Build history of the part. All positions in model axes, mm. Face numbers are marked on the shaded views. A direction names the side the tool comes from. Give positions to 0.01 mm unless a question says otherwise; leave off trailing zeros. Loops run counter-clockwise (first coordinate to the right, second up) from the corner with the lowest first, then second, coordinate; pieces in that order, holes last. Notation, with made-up numbers: (57, 10.5) -> (111, 10.5) arc R24 cw to (111, 28.5) -> close; hole circle Ø10 at (-26.5, 49.5). An arc over 180 degrees is marked (long way). Answer as a JSON object with one key per item and string values. Group by question number.
Q1. Two-plate mould, pull along Z, no slides. Class the marked faces 5, 6 and 7: pulls with the +Z half, pulls with the -Z half, needs draft (parallel to the pull), parting line crosses it, or undercut.
Q2. Band-saw the part on D-D, the plane y = 7.5. Write the cut outline in (x, z), plus the area to 3 significant figures.
Q3. Band-saw the part on A-A, the plane y = 23. Write the cut outline in (x, z).
Q4. Band-saw the part on C-C, the plane z = -8. Write the cut outline in (x, y).
Q5. Drop flat-ended pins along their axis: pin 1 (3 mm diameter, centred on y = 15.5, z = 6.5, fed in from -X); pin 2 (9 mm diameter, centred on x = 4, y = 13.5, fed in from -Z); pin 3 (3 mm diameter, centred on y = 9, z = -2, fed in from +X). Give the stop position or say it passes through.
Q6. Tool access for the marked faces 1, 2, 3 and 4: list every direction of +Z, -Z, +X, -X, +Y, -Y with a clear straight run to the whole face (end or side of a thin tool).
Q7. Band-saw the part on B-B, the plane x = 0. Write the cut outline in (y, z).
Q8. Wall check: probe 1 along Z at (x, y) = (-7.25, 7.5); probe 2 along Z at (x, y) = (0, 8.5); probe 3 along Z at (x, y) = (-8.5, 5). Give the ranges that are in metal, low to high. Write a range as from..to.
Autodesk Inventor part; units mm, degrees
ref_plane "РабПлоскость1" through (0, 0, 11.75) normal (0, 0, 1) x (1, 0, 0)
ref_plane "YZ Plane" through (0, 0, 0) normal (1, 0, 0) x (0, 1, 0)
ref_plane "XZ Plane" through (0, 0, 0) normal (0, 1, 0) x (-1, 0, 0)
sketch "Эскиз1" plane through (0, 0, 0) normal (0, 1, 0) x (-1, 0, 0)
  circle A0 centre (0, 0) radius 11.75
  dimension "d0" = 23.5
extrude "Выдавливание1" add sketch "Эскиз1" along normal blind 18
sketch "Эскиз2" plane through (0, 0, 0) normal (0, -1, 0) x (1, 0, 0)
  circle A0 centre (0, 0) radius 14
  dimension "d3" = 28
extrude "Выдавливание2" add sketch "Эскиз2" along normal blind 2
sketch "Эскиз3" plane through (0, 18, 0) normal (0, 1, 0) x (1, 0, 0)
  line L0 (0, 11.75) -> (0, -11.75) construction
  line L1 (-0.6, 11.7347) -> (-0.6, 2.4269)
  line L2 (0.6, 11.7347) -> (0.6, 2.4269)
  line L3 (-11.75, 0) -> (11.75, 0) construction
  line L4 (-0.6, -11.7347) -> (-0.6, -2.4269)
  line L5 (0.6, -11.7347) -> (0.6, -2.4269)
  arc A0 (-0.6, 2.4269) -> (-0.6, -2.4269) centre (0, 0) ccw
  arc A1 (0.6, -2.4269) -> (0.6, 2.4269) centre (0, 0) ccw
  circle A2 centre (0, 0) radius 11.75
  line L6 (-11.3865, 2.9) -> (-4.75, 2.9)
  line L7 (-4.75, 2.9) -> (-4.75, -2.9)
  line L8 (-4.75, -2.9) -> (-11.3865, -2.9)
  line L9 (-7.75, 1.9) -> (-5.75, 1.9)
  line L10 (-5.75, 1.9) -> (-5.75, -1.9)
  line L11 (-5.75, -1.9) -> (-7.75, -1.9)
  line L12 (-7.75, -1.9) -> (-7.75, 1.9)
  dimension "d7" = 1.2
  dimension "d8" = 2.5
  dimension "d12" = 5.8
  dimension "d13" = 7
  dimension "d14" = 1
  dimension "d15" = 1
  dimension "d16" = 1
  dimension "d17" = 2
extrude "Выдавливание3" add sketch "Эскиз3" along normal blind 7 contours A2 L2 A1 L5 L4 A0 L1 | L6 L7 L8 A2
sketch "Эскиз4" plane through (0, -2, 0) normal (0, -1, 0) x (1, 0, 0)
  circle A0 centre (0, 0) radius 10.5
  dimension "d18" = 21
extrude "Выдавливание4" cut sketch "Эскиз4" against normal blind 18
sketch "Эскиз5" plane through (0, 0, 0) normal (0, 1, 0) x (1, 0, 0)
  arc A0 (0.6, -11.7347) -> (0.6, 11.7347) centre (0, 0) ccw
  line L0 (11.7155, 0.9) -> (12.95, 0.9)
  line L1 (12.95, 0.9) -> (12.95, -0.9)
  line L2 (12.95, -0.9) -> (11.7155, -0.9)
  line L3 (0, 0) -> (19.973, 0) construction
  point P0 (11.75, 0)
  point P1 (11.75, 0)
  dimension "d21" = 1.8
  dimension "d22" = 1.2
extrude "Выдавливание5" add sketch "Эскиз5" along normal blind 8
chamfer "Фаска1" distance 1.7 angle 35 1 edges at (12.95, 8, 0) measured on face at (12.95, 2.6667, -0.3)
ref_plane "РабПлоскость1" through (0, 0, 11.75) normal (0, 0, 1) x (1, 0, 0)
sketch "Эскиз7" plane through (0, 0, 11.75) normal (0, 0, 1) x (1, 0, 0)
  line L0 (11.75, 18) -> (0.6, 18)
  line L1 (-0.6, 18) -> (-11.3865, 18)
  line L2 (0, 18) -> (4.5, 18)
  line L3 (4.5, 18) -> (4.5, 16)
  line L4 (4.5, 0) -> (0, 0)
  line L5 (14, 0) -> (-14, 0)
  line L6 (0.6, 18) -> (-0.6, 18) construction
  line L7 (0, 18) -> (0, 0) construction
  line L8 (4.5, 0) -> (9.9502, 2.6511)
  line L9 (10.613, 4.7144) -> (4.5, 16)
  arc A0 (9.9502, 2.6511) -> (10.613, 4.7144) centre (9.2941, 4) ccw
  line L10 (0, 18) -> (-4.5, 18)
  line L11 (-4.5, 18) -> (-4.5, 16)
  line L12 (-4.5, 0) -> (0, 0)
  line L13 (-4.5, 0) -> (-9.9502, 2.6511)
  line L14 (-10.613, 4.7144) -> (-4.5, 16)
  arc A1 (-10.613, 4.7144) -> (-9.9502, 2.6511) centre (-9.2941, 4) ccw
  point P0 (11, 4)
  dimension "d30" = 9
  dimension "d31" = 4
  dimension "d32" = 22
  dimension "d33" = 1.5
  dimension "d34" = 2
  dimension "d35" = 154.061
extrude "Выдавливание6" add sketch "Эскиз7" along normal mid plane 0.8
mirror "Зеркальное отражение1" about plane through (0, 0, 0) normal (0, 0, 1) of "Выдавливание6"
sketch "Эскиз9" plane through (0, 0, 12.15) normal (0, 0, 1) x (1, 0, 0)
  line L0 (4.5, 0) -> (-4.5, 0)
  line L1 (4.5, 0) -> (9.9502, 2.6511)
  arc A0 (9.9502, 2.6511) -> (10.613, 4.7144) centre (9.2941, 4) ccw
  line L2 (10.613, 4.7144) -> (4.5, 16)
  line L3 (4.5, 16) -> (4.5, 18)
  line L4 (4.5, 18) -> (-4.5, 18)
  line L5 (-4.5, 18) -> (-4.5, 16)
  line L6 (-4.5, 16) -> (-10.613, 4.7144)
  arc A1 (-10.613, 4.7144) -> (-9.9502, 2.6511) centre (-9.2941, 4) ccw
  line L7 (-9.9502, 2.6511) -> (-4.5, 0)
  line L8 (4.2, 5.25) -> (10.3229, 5.25)
  line L9 (10.1232, 2.75) -> (4.2, 2.75)
  line L10 (4.2, 2.75) -> (4.2, 5.25)
  line L11 (0, 18) -> (0, 0) construction
  line L12 (9.2941, 4) -> (-9.2941, 4) construction
  arc A2 (-10.613, 4.7144) -> (-9.9502, 2.6511) centre (-9.2941, 4) ccw
  line L13 (-4.2, 5.25) -> (-10.3229, 5.25)
  line L14 (-10.1232, 2.75) -> (-4.2, 2.75)
  line L15 (-4.2, 2.75) -> (-4.2, 5.25)
  dimension "d40" = 4.2
  dimension "d43" = 2.5
extrude "Выдавливание8" add sketch "Эскиз9" along normal blind 1.2 contours L9 L10 L8 L2 A0 | A1 L6 L13 L15 L14
chamfer "Фаска2" distance 2.05 angle 30 1 edges at (7.2615, 5.25, 13.35) measured on face at (8.2154, 4.4167, 13.35)
chamfer "Фаска3" distance 2.05 angle 30 1 edges at (-7.2615, 5.25, 13.35) measured on face at (-8.2154, 4.4167, 13.35)
mirror "Зеркальное отражение2" about plane through (0, 0, 0) normal (0, 0, 1) of "Выдавливание8", "Фаска2", "Фаска3"
equation "\"d15\" = d14"
equation "\"d16\" = d14"
properties material "Пластмасса, непрозрачная, черная"
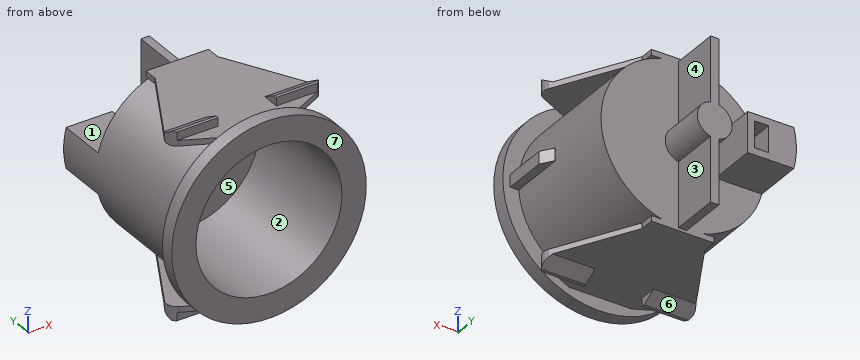
Worked answers:
{
 "1": {"face 5": "undercut", "face 6": "pulls with the -Z half", "face 7": "needs draft"},
 "2": {"outline": "(-9.1, -12.15) -> (9.1, -12.15) -> (9.1, -11.35) -> (3.04, -11.35) arc R11.75 ccw to (11.72, -0.9) -> (12.11, -0.9) -> (12.11, 0.9) -> (11.72, 0.9) arc R11.75 ccw to (3.04, 11.35) -> (9.1, 11.35) -> (9.1, 12.15) -> (-9.1, 12.15) -> (-9.1, 11.35) -> (-3.04, 11.35) arc R11.75 ccw to (-3.04, -11.35) -> (-9.1, -11.35) -> close; hole circle Ø21 at (0, 0)", "area": "114 mm2"},
 "3": {"outline": "(-11.39, -2.9) -> (-4.75, -2.9) -> (-4.75, 2.9) -> (-11.39, 2.9) arc R11.75 ccw to start; (-0.6, -11.73) arc R11.75 ccw to (0.6, -11.73) -> (0.6, -2.43) arc R2.5 ccw to (0.6, 2.43) -> (0.6, 11.73) arc R11.75 ccw to (-0.6, 11.73) -> (-0.6, 2.43) arc R2.5 ccw to (-0.6, -2.43) -> close; hole (-7.75, -1.9) -> (-5.75, -1.9) -> (-5.75, 1.9) -> (-7.75, 1.9) -> close"},
 "4": {"outline": "(-11.49, -2) -> (-6.8, -2) -> (-6.8, 16) -> (6.8, 16) -> (6.8, -2) -> (11.49, -2) -> (11.49, 0) -> (8.61, 0) -> (8.61, 18) -> (0.6, 18) -> (0.6, 25) -> (-0.6, 25) -> (-0.6, 18) -> (-8.61, 18) -> (-8.61, 0) -> (-11.49, 0) -> close"},
 "5": {"pin 1": "x = -10.63", "pin 2": "z = -12.15", "pin 3": "x = 11.77"},
 "6": {"face 1": "+Z, -X, +Y", "face 2": "-Y", "face 3": "-Z, +X, +Y", "face 4": "+Z, +X, +Y"},
 "7": {"outline": "(-2, -14) -> (0, -14) -> (0, -12.15) -> (18, -12.15) -> (18, -11.75) -> (25, -11.75) -> (25, 11.75) -> (18, 11.75) -> (18, 12.15) -> (0, 12.15) -> (0, 14) -> (-2, 14) -> (-2, 10.5) -> (16, 10.5) -> (16, -10.5) -> (-2, -10.5) -> close"},
 "8": {"probe 1": "-12.15..-11.35, -9.25..-7.6, 7.6..9.25, 11.35..12.15", "probe 2": "-12.15..-10.5, 10.5..12.15", "probe 3": "-12.31..-11.35, -8.11..-6.16, 6.16..8.11, 11.35..12.31"}
}
